```python
from build123d import *

# Parameters (mm, degrees)
SKETCH1_W                = 110
SKETCH1_H                = 90
BOSS_EXTRUDE1_DEPTH      = 6
SKETCH2_W                = 25
SKETCH2_H                = 10
CUT_EXTRUDE1_DEPTH       = 7
MIRROR2_COPY_1_SKETCH_W  = 25
MIRROR2_COPY_1_SKETCH_H  = 10
MIRROR2_COPY_1_DEPTH     = 7
M3_CLEARANCE_HOLE1_D     = 3.2
M3_CLEARANCE_HOLE2_D     = 3.2
FILLET1_R                = 5
SKETCH62_W               = 10
SKETCH62_H               = 6
CUT_EXTRUDE12_DEPTH      = 4
CUT_EXTRUDE12_DEPTH_BACK = 4


with BuildPart() as part:
    # Sketch1 → Boss-Extrude1 (new body)
    with BuildSketch(Plane(origin=(0, 0, 0), x_dir=(1, 0, 0), z_dir=(0, 1, 0))):
        Rectangle(SKETCH1_W, SKETCH1_H)
    extrude(amount=BOSS_EXTRUDE1_DEPTH)

    # Sketch2 → Cut-Extrude1 (cut, through all)
    with BuildSketch(Plane(origin=(0, 6, 0), x_dir=(1, 0, 0), z_dir=(0, 1, 0))):
        with Locations((30, 30)):
            Rectangle(SKETCH2_W, SKETCH2_H)
    cut_extrude1 = extrude(amount=-CUT_EXTRUDE1_DEPTH, mode=Mode.SUBTRACT)

    # Mirror1: Cut-Extrude1 across plane
    add(cut_extrude1.mirror(Plane.XY), mode=Mode.SUBTRACT)

    # Mirror2: Cut-Extrude1 across plane
    add(cut_extrude1.mirror(Plane(origin=(0, 0, 0), x_dir=(0, 0, 1), z_dir=(1, 0, 0))), mode=Mode.SUBTRACT)

    # Mirror2 copy 1 sketch → Mirror2 copy 1 (cut, through all)
    with BuildSketch(Plane(origin=(0, 6, 0), x_dir=(-1, 0, 0), z_dir=(0, 1, 0))):
        with Locations((30, 30)):
            Rectangle(MIRROR2_COPY_1_SKETCH_W, MIRROR2_COPY_1_SKETCH_H)
    extrude(amount=-MIRROR2_COPY_1_DEPTH, mode=Mode.SUBTRACT)

    # M3 Clearance Hole1 (through all)
    with Locations(Plane(origin=(0, 6, 0), x_dir=(1, 0, 0), z_dir=(0, 1, 0))):
        with Locations((17.5, 15), (37.5, 15), (17.5, -15), (37.5, -15)):
            Hole(M3_CLEARANCE_HOLE1_D / 2)

    # M3 Clearance Hole2 (through all)
    with Locations(Plane(origin=(0, 6, 0), x_dir=(1, 0, 0), z_dir=(0, 1, 0))):
        with Locations((48.75, 40), (0, 40), (-48.75, 40), (-48.75, -40), (0, -40), (48.75, -40), (-10, 0)):
            Hole(M3_CLEARANCE_HOLE2_D / 2)

    # Fillet1
    fillet1_edges = [part.edges().sort_by_distance(p)[0] for p in [
        (55, 3, 45),
        (-55, 3, 45),
        (-55, 3, -45),
        (55, 3, -45),
    ]]
    fillet(fillet1_edges, radius=FILLET1_R)

    # Sketch62 → Cut-Extrude12 (cut, two sides)
    with BuildSketch(Plane(origin=(-39.232221392, 3, -44.54), x_dir=(-1, 0, 0), z_dir=(0, -1, 0))) as cut_extrude12_sk:
        with Locations((0.767778608, -44)):
            Rectangle(SKETCH62_W, SKETCH62_H)
    extrude(amount=CUT_EXTRUDE12_DEPTH, mode=Mode.SUBTRACT)
    extrude(cut_extrude12_sk.sketch, amount=-CUT_EXTRUDE12_DEPTH_BACK, mode=Mode.SUBTRACT)


solid = part.part
```
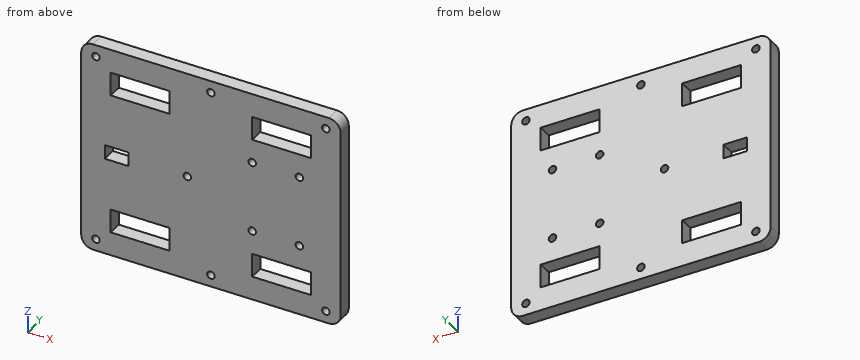
Geometry: final body of the model. Coordinates: model frame, mm. Round coordinates to 2 decimals unless told otherwise and drop trailing zeros. Order: outer loops, then holes, each group sorted by start corner. A loop starts at its lowest first (then second) coordinate and runs counter-clockwise, first axis right, second up. Notation, with made-up numbers: (-10, 15.25) -> (6, 15.25) arc R12 cw to (6, 34.25) -> close; hole circle Ø11 at (1.25, 54). An arc over 180 degrees is marked (long way). Use CSV: the item, a comma, the result in double quotes. Start each with the question number.
1) Section C-C (x = 37.5). Return the cut outline in (y, z).
2) Section B-B (x = 48.75). Return the cut outline in (y, z).
3) Section D-D (y = 2.2). State how many separate pieces and enclosed holes the cut face has, and give its area (3 significant figures).
4) Section A-A (z = -15). Return the cut outline in (x, y).
5) Material intervals for line 1 along X through (y, z) = (4.6, 15); line 2 along Z through (x, y) = (-28, 1.1); line 3 along X through (y, z) = (0.7, -30), sorted ascending. Write a range as from..to.
Returned:
1,outline,"(0, -45) -> (6, -45) -> (6, -35) -> (0, -35) -> close; (0, -25) -> (6, -25) -> (6, -16.6) -> (0, -16.6) -> close; (0, -13.4) -> (6, -13.4) -> (6, 13.4) -> (0, 13.4) -> close; (0, 16.6) -> (6, 16.6) -> (6, 25) -> (0, 25) -> close; (0, 35) -> (6, 35) -> (6, 45) -> (0, 45) -> close"
2,outline,"(0, -45) -> (6, -45) -> (6, -41.6) -> (0, -41.6) -> close; (0, -38.4) -> (6, -38.4) -> (6, 38.4) -> (0, 38.4) -> close; (0, 41.6) -> (6, 41.6) -> (6, 45) -> (0, 45) -> close"
3,separate pieces,"1"
3,enclosed holes,"16"
3,area,"8,730 mm²"
4,outline,"(-55, 0) -> (15.9, 0) -> (15.9, 6) -> (-55, 6) -> close; (19.1, 0) -> (35.9, 0) -> (35.9, 6) -> (19.1, 6) -> close; (39.1, 0) -> (55, 0) -> (55, 6) -> (39.1, 6) -> close"
5,line 1,"x = -55..15.9, 19.1..35.9, 39.1..55"
5,line 2,"z = -45..-35, -25..25, 35..45"
5,line 3,"x = -55..-42.5, -17.5..17.5, 42.5..55"
